Input: part model. Units: mm. Frame: model coordinates. Give positions to 0.01 mm unless a question says otherwise; leave off trailing zeros. Loops run counter-clockwise (first coordinate to the right, second up) from the corner with the lowest first, then second, coordinate; pieces in that order, holes last. Notation, with made-up numbers: M 71.5,29 L 88.5,29 A25 ccw 88.5,57 Z; hole C -5.5,49.5 d9. An arc over 180 degrees is marked long. One line per item, written item: value. Start each with the question number.
(1) Ray query, line 1 along X through (y, z) = (21, 0); line 2 along Z through (x, y) = (-3.25, 19.25); line 3 along Y through (x, z) = (1.25, 4.25). Return the intervals inside material, ascending. Write a range as from..to.
(2) Section A-A on z = 0. Output: boundary loops of the cut face in (x, y), plus the area to 3 significant figures.
(3) Section C-C on y = 17. Output: boundary loops of the cut face in (x, z), plus the area to 3 significant figures.
(4) Section B-B on x = 0. Output: boundary loops of the cut face in (y, z).
(5) Pin query (flat end, axial travel): P1, Ø9, axis at x = 0, z = 0, coming from the -Y side. Return the tip coordinate at first contact, or that it passes through.
(6) Pull-direction query (Z, two-part tool) for faces 1 (the cylindrical face through (0.196, 29.699, 14.715)), 2 (the cylindrical face through (14.699, 29.715, -0.196)), 3 (the cylindrical face through (0.196, 0.301, -14.715)), 4 (the cylindrical face through (-3.905, 15.196, -0.867)); classes: released by +Z, released by -Z, zero draft, split by the parting line, or undercut.
```python
from build123d import *

# Parameters (mm, degrees)
SKIZZE1_W                       = 30
SKIZZE1_H                       = 30
AUFSATZ_LINEAR_AUSTRAGEN1_DEPTH = 30
SKIZZE2_R                       = 4
SCHNITT_LINEAR_AUSTRAGEN1_DEPTH = 31
VERRUNDUNG1_R                   = 1


with BuildPart() as part:
    # Skizze1 → Aufsatz-Linear austragen1 (new body)
    with BuildSketch(Plane(origin=(0, 0, 0), x_dir=(1, 0, 0), z_dir=(0, 1, 0))):
        Rectangle(SKIZZE1_W, SKIZZE1_H)
    extrude(amount=AUFSATZ_LINEAR_AUSTRAGEN1_DEPTH)

    # Skizze2 → Schnitt-Linear austragen1 (cut)
    with BuildSketch(Plane(origin=(0, 30, 0), x_dir=(1, 0, 0), z_dir=(0, 1, 0))):
        with Locations(Location((0, 0, 0), (0, 0, 270))):
            Circle(SKIZZE2_R)
    extrude(amount=-SCHNITT_LINEAR_AUSTRAGEN1_DEPTH, mode=Mode.SUBTRACT)

    # Verrundung1
    verrundung1_edges = [part.edges().sort_by_distance(p)[0] for p in [
        (-15, 30, 0),
        (0, 0, -4),
        (0, 30, -4),
        (0, 30, 15),
        (15, 30, 0),
        (0, 0, 15),
        (-15, 0, 0),
        (0, 0, -15),
        (15, 0, 0),
        (15, 15, 15),
        (-15, 15, 15),
        (-15, 15, -15),
        (15, 15, -15),
        (0, 30, -15),
    ]]
    fillet(verrundung1_edges, radius=VERRUNDUNG1_R)


solid = part.part
```
Output values:
1. line 1: x = -15..-4, 4..15
1. line 2: z = -15..-2.33, 2.33..15
1. line 3: y = 0.18..29.82
2. outline: M -15,1 A1 ccw -14,0 L -5,0 A1 ccw -4,1 L -4,29 A1 ccw -5,30 L -14,30 A1 ccw -15,29 Z; M 4,1 A1 ccw 5,0 L 14,0 A1 ccw 15,1 L 15,29 A1 ccw 14,30 L 5,30 A1 ccw 4,29 Z
2. area: 658 mm²
3. outline: M -15,-14 A1 ccw -14,-15 L 14,-15 A1 ccw 15,-14 L 15,14 A1 ccw 14,15 L -14,15 A1 ccw -15,14 Z; hole C 0,0 d8
3. area: 849 mm²
4. outline: M 0,-14 A1 ccw 1,-15 L 29,-15 A1 ccw 30,-14 L 30,-5 A1 ccw 29,-4 L 1,-4 A1 ccw 0,-5 Z; M 0,5 A1 ccw 1,4 L 29,4 A1 ccw 30,5 L 30,14 A1 ccw 29,15 L 1,15 A1 ccw 0,14 Z
5. P1: stops at y = 0.13
6. face 1: released by +Z
6. face 2: zero draft
6. face 3: released by -Z
6. face 4: undercut
